from build123d import *

# Parameters (mm, degrees)
CROQUIS1_W              = 120
CROQUIS1_H              = 100
SALIENTE_EXTRUIR1_DEPTH = 3
CROQUIS2_R              = 2
CROQUIS2_R_2            = 3.5
CORTAR_EXTRUIR1_DEPTH   = 3
CROQUIS3_W              = 120
CROQUIS3_H              = 100
CROQUIS3_W_2            = 114
CROQUIS3_H_2            = 94
SALIENTE_EXTRUIR2_DEPTH = 25


with BuildPart() as part:
    # Croquis1 → Saliente-Extruir1 (new body)
    with BuildSketch(Plane.XY):
        with Locations((60, 50)):
            Rectangle(CROQUIS1_W, CROQUIS1_H)
    extrude(amount=SALIENTE_EXTRUIR1_DEPTH)

    # Croquis2 → Cortar-Extruir1 (cut)
    with BuildSketch(Plane.XY.offset(3)):
        Polygon((11, 80), (11, 60), (11, 40), (109, 40), (109, 80), align=None)
        with Locations((13.5, 87.5)):
            Circle(CROQUIS2_R)
        with Locations((106.5, 87.5)):
            Circle(CROQUIS2_R)
        with Locations((106.5, 32.5)):
            Circle(CROQUIS2_R)
        with Locations((13.5, 32.5)):
            Circle(CROQUIS2_R)
        with Locations((30, 22)):
            Circle(CROQUIS2_R_2)
        with Locations((60, 22)):
            Circle(CROQUIS2_R_2)
        with Locations((90, 22)):
            Circle(CROQUIS2_R_2)
    extrude(amount=-CORTAR_EXTRUIR1_DEPTH, mode=Mode.SUBTRACT)

    # Croquis3 → Saliente-Extruir2 (add)
    with BuildSketch(Plane.XY.offset(3)):
        with Locations((60, 50)):
            Rectangle(CROQUIS3_W, CROQUIS3_H)
        with Locations((60, 50)):
            Rectangle(CROQUIS3_W_2, CROQUIS3_H_2, mode=Mode.SUBTRACT)
    extrude(amount=SALIENTE_EXTRUIR2_DEPTH)


solid = part.part
The listing builds one solid part. Answer for the finished solid, in the listing's coordinates (mm). A direction names the side the tool comes from. Coordinates: 2 decimals unless noted, no trailing zeros. Order: outer loops, then holes, each group sorted by start corner. A loop starts at its lowest first (then second) coordinate and runs counter-clockwise, first axis right, second up.
Q1. A cutting plane is placed at B-B, the plane x = 60. Write down the section's boundary in (y, z), and give its area (3 significant figures).
Q2. A cutting plane is placed at D-D, the plane x = 76.5. Write down the section's boundary in (y, z), and give its area (3 significant figures).
Q3. A cutting plane is placed at C-C, the plane y = 87.5. Write down the section's boundary in (x, z), and give its area (3 significant figures).
Q4. Consider line 1 (Y direction, x = 90, z = 0.7); line 2 (Y direction, x = 106.5, z = 1.85); line 3 (Y direction, x = 25, z = 26). Determine where each line is inside the solid, lowest interval first.
Q5. Given P1, Ø5.5, axis at x = 90, y = 22, coming from the +Z side; P2, Ø5, axis at x = 12, y = 22.5, coming from the +Z side, each flat-ended and moving along its own axis, determine where each tip first touches the part or whether it passes through.
Q6. A cutting plane is placed at A-A, the plane y = 22. Write down the section's boundary in (x, z).
Q7. Which of the six approach directions +Z, -Z, +X, -X, +Y, -Y give full straight-line access (tool end or side, diameter ignored) to faces 1 (the face through (117, 49, 15)), 2 (the face through (59, 40, 2)), 3 (the face through (120, 49, 14))?
Q8. For a pull along Y with two mould halves and no side action, classify faces 4 (the face through (0, 49, 14)), 5 (the face through (13.066, 30.548, 1.521)), 6 (the face through (59, 0, 14)) as pulls with the +Y half, pulls with the -Y half, needs draft (parallel to the pull), parting line crosses it, or undercut.
Answers follow:
1. outline: (0, 0) - (18.5, 0) - (18.5, 3) - (3, 3) - (3, 28) - (0, 28) - close; (25.5, 0) - (40, 0) - (40, 3) - (25.5, 3) - close; (80, 0) - (100, 0) - (100, 28) - (97, 28) - (97, 3) - (80, 3) - close
1. area: 309 mm2
2. outline: (0, 0) - (40, 0) - (40, 3) - (3, 3) - (3, 28) - (0, 28) - close; (80, 0) - (100, 0) - (100, 28) - (97, 28) - (97, 3) - (80, 3) - close
2. area: 330 mm2
3. outline: (0, 0) - (11.5, 0) - (11.5, 3) - (3, 3) - (3, 28) - (0, 28) - close; (15.5, 0) - (104.5, 0) - (104.5, 3) - (15.5, 3) - close; (108.5, 0) - (120, 0) - (120, 28) - (117, 28) - (117, 3) - (108.5, 3) - close
3. area: 486 mm2
4. line 1: y = 0 to 18.5, 25.5 to 40, 80 to 100
4. line 2: y = 0 to 30.5, 34.5 to 40, 80 to 85.5, 89.5 to 100
4. line 3: y = 0 to 3, 97 to 100
5. P1: passes through
5. P2: stops at z = 3
6. outline: (0, 0) - (26.5, 0) - (26.5, 3) - (3, 3) - (3, 28) - (0, 28) - close; (33.5, 0) - (56.5, 0) - (56.5, 3) - (33.5, 3) - close; (63.5, 0) - (86.5, 0) - (86.5, 3) - (63.5, 3) - close; (93.5, 0) - (120, 0) - (120, 28) - (117, 28) - (117, 3) - (93.5, 3) - close
7. face 1: +Z
7. face 2: +Z, -Z
7. face 3: +Z, -Z, +X, +Y, -Y
8. face 4: needs draft
8. face 5: undercut
8. face 6: pulls with the -Y half
